Check sheet for the modelled part. Datum: model origin and axes. Units: mm. A direction names the side the tool comes from. Round coordinates to 2 decimals unless told otherwise and drop trailing zeros. Loops run counter-clockwise (first coordinate to the right, second up) from the corner with the lowest first, then second, coordinate; pieces in that order, holes last. Notation, with made-up numbers: M 7,75.5 L 54,75.5 A18 ccw 54,104.5 Z; hole C -26,63.25 d10. An arc over 180 degrees is marked long. One line per question, with ' | ' between items. Start each with the question number.
(1) Tool access check on faces 1 (the face through (5, 19.5, 5)), 2 (the face through (22.7, -34.5, 4.9)), 3 (the face through (10, -27, 5)). Record the directions out of +Z, -Z, +X, -X, +Y, -Y that give a thin tool (end or side, any length) a straight path to the whole face; none if there is none.
(2) Go/stop test with flat-tipped pins: P1, Ø1, axis at y = -17.5, z = 6, coming from the +X side; P2, Ø2, axis at x = 17, z = 6.5, coming from the -Y side; P3, Ø3, axis at y = 24, z = 4, coming from the -X side. Record where each tip stops, or that it passes through.
(3) Section check D-D (x = 15). Record the boundary of the cut face in (y, z), and give its area (3 significant figures).
(4) Thickness scan on probe 1 along Y at (x, z) = (5, 7); probe 2 along X at (y, z) = (-5, 5.25); probe 3 along Y at (x, z) = (24, 9.5). Record the ranges inside material, lowest first. Write a range as [from, to].
(5) Section check B-B (x = 9). Record the boundary of the cut face in (y, z).
```python
from build123d import *

# Parameters (mm, degrees)
BOSS_EXTRUDE1_DEPTH = 10
FILLET1_R           = 5
FILLET2_R           = 5


# Some blends are built 0.0001 mm under size
with BuildPart() as part:
    # Sketch1 → Boss-Extrude1 (new body)
    with BuildSketch(Plane.XY):
        Polygon((0, -19.5), (0, 19.5), (10, 19.5), (10, 34.5), (40, 34.5), (40, -34.5), (10, -34.5), (10, -19.5), align=None)
    extrude(amount=BOSS_EXTRUDE1_DEPTH)

    # Fillet1
    fillet1_edges = [part.edges().sort_by_distance(p)[0] for p in [
        (40, 0, 10),
        (40, 34.5, 5),
        (40, -34.5, 5),
        (40, 0, 0),
    ]]
    fillet(fillet1_edges, radius=FILLET1_R - 0.0001)  # a hair under: the kernel refuses the full size

    # Fillet2
    # the kernel refuses this fillet: 5 mm, written as the material it takes off along each edge
    with BuildSketch(Plane(origin=(40, 29.5, 5), x_dir=(0, 0, -1), z_dir=(0, -1, 0))) as fillet2_piece_1:
        with BuildLine():
            CenterArc((0.0001, -4.9999), 4.9999, 0, 90)
            Line((5, -4.9999), (5, 0))
            Line((5, 0), (0.0001, 0))
        make_face()
    revolve(axis=Axis((40, 29.5, 5), (1, 0, 0)), revolution_arc=90, mode=Mode.SUBTRACT)
    with BuildSketch(Plane(origin=(40, 29.5, 5), x_dir=(0, 1, 0), z_dir=(0, 0, -1))) as fillet2_piece_2:
        with BuildLine():
            CenterArc((0.0001, -4.9999), 4.9999, 0, 90)
            Line((5, -4.9999), (5, 0))
            Line((5, 0), (0.0001, 0))
        make_face()
    revolve(axis=Axis((40, 29.5, 5), (1, 0, 0)), revolution_arc=90, mode=Mode.SUBTRACT)
    with BuildSketch(Plane(origin=(40, -29.5, 5), x_dir=(0, -1, 0), z_dir=(0, 0, 1))) as fillet2_piece_3:
        with BuildLine():
            CenterArc((0.0001, -4.9999), 4.9999, 0, 90)
            Line((5, -4.9999), (5, 0))
            Line((5, 0), (0.0001, 0))
        make_face()
    revolve(axis=Axis((40, -29.5, 5), (1, 0, 0)), revolution_arc=90, mode=Mode.SUBTRACT)
    with BuildSketch(Plane(origin=(40, -29.5, 5), x_dir=(0, 0, 1), z_dir=(0, 1, 0))) as fillet2_piece_4:
        with BuildLine():
            CenterArc((0.0001, -4.9999), 4.9999, 0, 90)
            Line((5, -4.9999), (5, 0))
            Line((5, 0), (0.0001, 0))
        make_face()
    revolve(axis=Axis((40, -29.5, 5), (1, 0, 0)), revolution_arc=90, mode=Mode.SUBTRACT)
    with BuildSketch(Plane(origin=(-2.5, 34.5, 0), x_dir=(0, 0, 1), z_dir=(1, 0, 0)), Plane(origin=(40, -34.5, 10), x_dir=(0, 1, 0), z_dir=(-1, 0, 0))) as fillet2_piece_5:
        with BuildLine():
            CenterArc((FILLET2_R, FILLET2_R), FILLET2_R, 180, 90)
            Line((0, FILLET2_R), (0, 0))
            Line((0, 0), (FILLET2_R, 0))
        make_face()
    extrude(amount=42.5, mode=Mode.SUBTRACT)
    with BuildSketch(Plane(origin=(-2.5, 34.5, 10), x_dir=(0, 0, -1), z_dir=(1, 0, 0)), Plane(origin=(40, -34.5, 0), x_dir=(0, 1, 0), z_dir=(-1, 0, 0))) as fillet2_piece_6:
        with BuildLine():
            CenterArc((FILLET2_R, -FILLET2_R), FILLET2_R, 90, 90)
            Line((0, -FILLET2_R), (0, 0))
            Line((0, 0), (FILLET2_R, 0))
        make_face()
    extrude(amount=42.5, mode=Mode.SUBTRACT)


solid = part.part
```
The answers:
1) face 1: +Z, -Z, -X, +Y | face 2: +X, -X, -Y | face 3: +Z, -Z, -X, -Y
2) P1: x = 39.97 | P2: y = -34.47 | P3: x = 10
3) outline: M -29.5,0 L 29.5,0 A5 ccw 29.5,10 L -29.5,10 A5 ccw Z | area: 669 mm²
4) probe 1: [-19.5, 19.5] | probe 2: [0, 39.99] | probe 3: [-31.68, 31.68]
5) outline: M -19.5,0 L 19.5,0 L 19.5,10 L -19.5,10 Z
